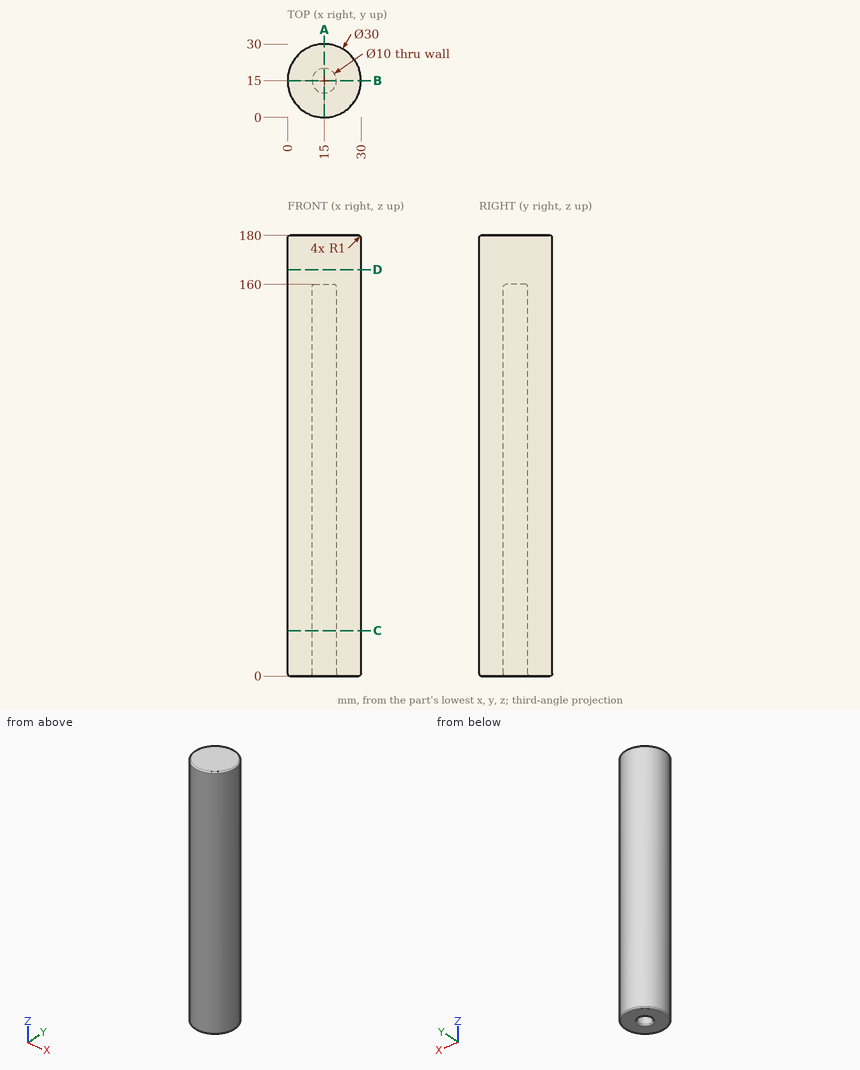
Geometry: see drawing. Coordinates: mm, zero at the bounding-box minimum. Round coordinates to 2 decimals unless told otherwise and drop trailing zeros. Write each loop counter-clockwise with the first axis right and the second up, starting at its lowest first coordinate (ties: lowest second). Pieces come first, ordered by that corner, then holes.
Item 1: Pin query (flat end, axial travel): P1, Ø5, axis at x = 8.5, z = 96, coming from the +Y side; P2, Ø2, axis at y = 24.5, z = 139.5, coming from the -X side; P3, Ø4, axis at x = 15, y = 13.5, coming from the -Z side. Return the tip coordinate at first contact, or that it passes through.
Item 2: Section query A-A (x = 15). Return loops of the section in (y, z).
Item 3: Material intervals for L1, parallel to Y at x = 15, z = 76; L2, parallel to X at y = 19.5, z = 14; L3, parallel to Y at x = 14, z = 27.5, sorted ascending.
Item 4: Section query C-C (z = 18.5). Return loops of the section in (x, y).
Item 5: Section query D-D (z = 166). Return loops of the section in (x, y).
Completed:
1. P1: stops at y = 29.46
1. P2: stops at x = 2.64
1. P3: stops at z = 160
2. outline: (0, 1) arc R1 ccw to (1, 0) - (9, 0) arc R1 ccw to (10, 1) - (10, 159) arc R1 cw to (11, 160) - (19, 160) arc R1 cw to (20, 159) - (20, 1) arc R1 ccw to (21, 0) - (29, 0) arc R1 ccw to (30, 1) - (30, 179) arc R1 ccw to (29, 180) - (1, 180) arc R1 ccw to (0, 179) - close
3. L1: y = 0 to 10, 20 to 30
3. L2: x = 0.69 to 12.82, 17.18 to 29.31
3. L3: y = 0.03 to 10.1, 19.9 to 29.97
4. outline: circle Ø30 at (15, 15); hole circle Ø10 at (15, 15)
5. outline: circle Ø30 at (15, 15)
